For this review, use the dimensioned drawing (mm, ordinates from the lowest corner) and the shaded views. Round coordinates to 2 decimals unless told otherwise and drop trailing zeros. Write each loop counter-clockwise with the first axis right and the second up, starting at its lowest first coordinate (ties: lowest second). Pieces come first, ordered by that corner, then holes. Notation, with made-up numbers: (31, 46) - (77, 46) arc R23 ccw to (77, 81) - close; hole circle Ø11 at (13.25, 2.5). An arc over 180 degrees is marked (long way). Write each question's results on one line, items separated by ' | '.
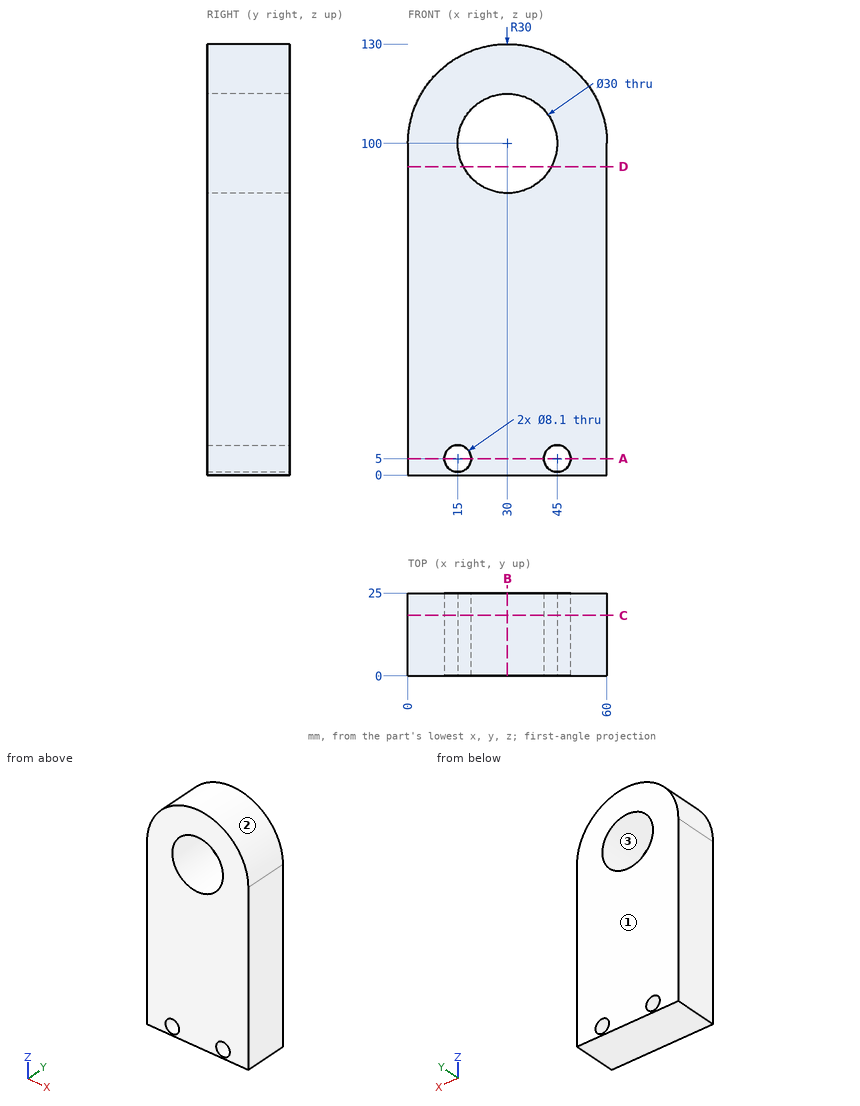
Q1. Insertion check: P1, Ø10, axis at y = 18.5, z = 114, coming from the -X side; P2, Ø2, axis at y = 7.5, z = 18, coming from the -X side; P3, Ø7.5, axis at x = 45, z = 5, coming from the -Y side. Each pin has a flat end and moves straight along its axis. Give the tip position at first contact, or say it passes through.
Evaluation:
P1: stops at x = 1.38 | P2: stops at x = 0 | P3: passes through
Q2. We need section A-A (z = 5). State the section outline as (x, y) points.
Evaluation:
outline: (0, 0) - (10.95, 0) - (10.95, 25) - (0, 25) - close; (19.05, 0) - (40.95, 0) - (40.95, 25) - (19.05, 25) - close; (49.05, 0) - (60, 0) - (60, 25) - (49.05, 25) - close
Q3. For probe 1 along X at (y, z) = (14.25, 5); probe 2 along Z at (x, y) = (30, 16.5); probe 3 along Z at (x, y) = (18.5, 6), list the stretches that pass through material, from the lowest coordinate up.
Evaluation:
probe 1: x = 0 to 10.95, 19.05 to 40.95, 49.05 to 60 | probe 2: z = 0 to 85, 115 to 130 | probe 3: z = 0 to 2.96, 7.04 to 90.37, 109.63 to 127.71
Q4. We need section D-D (z = 93). State the section outline as (x, y) points, plus the area to 3 significant figures.
Evaluation:
outline: (0, 0) - (16.73, 0) - (16.73, 25) - (0, 25) - close; (43.27, 0) - (60, 0) - (60, 25) - (43.27, 25) - close | area: 837 mm^2
Q5. The part is to be moulded in two halves that separate along Z. For the marked faces 1, 2 and 3, say which applies: released by +Z, released by -Z, zero draft, split by the parting line, or undercut.
Evaluation:
face 1: zero draft | face 2: released by +Z | face 3: undercut
Q6. We need section C-C (y = 18.25). State the section outline as (x, z) points.
Evaluation:
outline: (0, 0) - (60, 0) - (60, 100) arc R30 ccw to (0, 100) - close; hole circle Ø8.1 at (15, 5); hole circle Ø30 at (30, 100); hole circle Ø8.1 at (45, 5)
Q7. We need section B-B (x = 30). State the section outline as (y, z) points.
Evaluation:
outline: (0, 0) - (25, 0) - (25, 85) - (0, 85) - close; (0, 115) - (25, 115) - (25, 130) - (0, 130) - close
